```python
from build123d import *

# Parameters (mm, degrees)
F0_W        = 88.9
F0_H        = 38.1
F1_DEPTH    = 25.4
F2_T1_DEPTH = 152.4
F2_T3_DEPTH = 215.9


# Not quite as in the source:
# - a fillet or chamfer that OpenCascade refuses, or shapes differently, is made with other operations: its cross-section is extruded or revolved along the edge and cut away or added


with BuildPart() as f1:
    # F0 (on Front) → F1 (new body)
    with BuildSketch(Plane.XZ):
        Rectangle(F0_W, F0_H)
    extrude(amount=F1_DEPTH)

    # F2: fillet of radius 25.4 on 4 edges, made by hand

    # F2_s2 → F2_t1 (cut)
    with BuildSketch(Plane.XZ.offset(-63.5)):
        with BuildLine():
            ThreePointArc((44.45, 6.35), (37.0105122421, -11.6105122421), (19.05, -19.05))
            Line((19.05, -19.05), (44.45, -19.05))
            Line((44.45, -19.05), (44.45, 6.35))
        make_face()
        with BuildLine():
            ThreePointArc((-44.45, 6.35), (-37.0105122421, -11.6105122421), (-19.05, -19.05))
            Line((-19.05, -19.05), (-44.45, -19.05))
            Line((-44.45, -19.05), (-44.45, 6.35))
        make_face()
    extrude(amount=F2_T1_DEPTH, mode=Mode.SUBTRACT)

    # F2_s4 → F2_t3 (cut)
    with BuildSketch(Plane.YZ.offset(-107.95)):
        with BuildLine():
            ThreePointArc((0, -19.05), (-17.9605122421, -11.6105122421), (-25.4, 6.35))
            Line((-25.4, 6.35), (-25.4, -19.05))
            Line((-25.4, -19.05), (0, -19.05))
        make_face()
        with BuildLine():
            ThreePointArc((-25.4, -19.05), (-7.4394877579, -11.6105122421), (0, 6.35))
            Line((0, 6.35), (0, -19.05))
            Line((0, -19.05), (-25.4, -19.05))
        make_face()
    extrude(amount=F2_T3_DEPTH, mode=Mode.SUBTRACT)


solid = f1.part
```
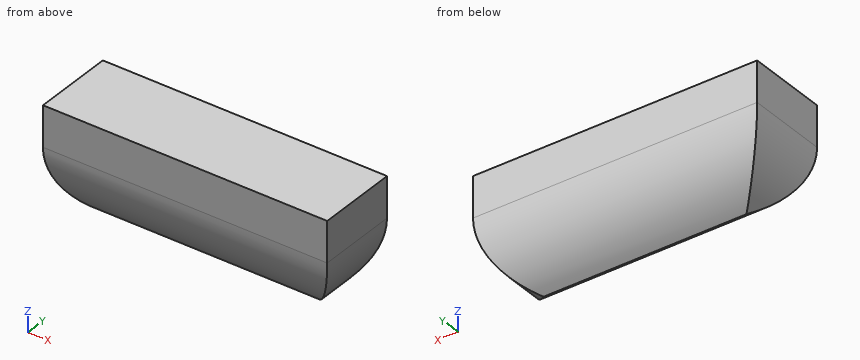
Model file for the job. Use its own axes, mm. Give positions to 0.01 mm unless a question says otherwise; leave off trailing zeros. Order: outer loops, then holes, each group sorted by start corner. A loop starts at its lowest first (then second) coordinate and runs counter-clockwise, first axis right, second up.
1) Saw through at A-A, the plane x = -17. Write the cut outline in (y, z), then the cut area to 3 significant figures.
2) Wall check: probe 1 along Y at (x, z) = (16.5, -7.5); probe 2 along Z at (x, y) = (-17.5, -19); probe 3 along Z at (x, y) = (-21, -6). Give the ranges that are in metal, low to high.
3) Saw through at C-C, the plane z = -12.5. Write the cut outline in (x, y), then the cut area to 3 significant figures.
4) Saw through at D-D, the plane y = -10. Write the cut outline in (x, z), then the cut area to 3 significant figures.
5) Pin check, flat tips, straight feed: pin 1 (3 mm diameter, centred on x = 19, y = -4, fed in from -Z); pin 2 (4 mm diameter, centred on x = -1, z = -7.5, fed in from -Y); pin 3 (10 mm diameter, centred on x = 2, z = -8, fed in from -Y). Stop position of each tip, or through.
6) Saw through at B-B, the plane y = -5.5. Write the cut outline in (x, z).
Computed:
1. outline: (-25.4, 6.35) arc R25.4 ccw to (-12.7, -15.65) arc R25.4 ccw to (0, 6.35) - (0, 19.05) - (-25.4, 19.05) - close
1. area: 719 mm2
2. probe 1: y = -21.29 to -4.11
2. probe 2: z = -10.51 to 19.05
2. probe 3: z = -10.05 to 19.05
3. outline: (-36.07, -17.02) - (36.07, -17.02) - (36.07, -8.38) - (-36.07, -8.38) - close
3. area: 624 mm2
4. outline: (-44.45, 6.35) arc R25.4 ccw to (-34.45, -13.85) - (34.45, -13.85) arc R25.4 ccw to (44.45, 6.35) - (44.45, 19.05) - (-44.45, 19.05) - close
4. area: 2,800 mm2
5. pin 1: stops at z = -9.43
5. pin 2: stops at y = -22.47
5. pin 3: stops at y = -23.62
6. outline: (-44.45, 6.35) arc R25.4 ccw to (-38.95, -9.43) - (38.95, -9.43) arc R25.4 ccw to (44.45, 6.35) - (44.45, 19.05) - (-44.45, 19.05) - close
